Check sheet for the modelled part. Datum: model origin and axes. Units: mm. Round coordinates to 2 decimals unless told otherwise and drop trailing zeros. Order: outer loops, then holes, each group sorted by start corner. A loop starts at its lowest first (then second) coordinate and runs counter-clockwise, first axis right, second up. Notation, with made-up numbers: (-38, 20) -> (-29, 20) arc R18 cw to (-29, 52) -> close; hole circle Ø9 at (-9, 4). An arc over 180 degrees is marked (long way). Answer in a Markdown table with one row per item.
from build123d import *

# Parameters (mm, degrees)
F1_DEPTH = 8


with BuildPart() as f1:
    # F0 (on Top) → F1 (new body)
    with BuildSketch(Plane.XY):
        with BuildLine():
            Line((24.033267, 22.719095), (12.033267, 22.719095))
            ThreePointArc((12.033267, 22.719095), (10.619054, 22.133308), (10.033267, 20.719095))
            Line((10.033267, 20.719095), (10.033267, 9.719095))
            ThreePointArc((10.033267, 9.719095), (10.619054, 8.304881), (12.033267, 7.719095))
            Line((12.033267, 7.719095), (24.033267, 7.719095))
            ThreePointArc((24.033267, 7.719095), (25.447481, 8.304881), (26.033267, 9.719095))
            Line((26.033267, 9.719095), (26.033267, 20.719095))
            ThreePointArc((26.033267, 20.719095), (25.447481, 22.133308), (24.033267, 22.719095))
        make_face()
        with BuildLine():
            ThreePointArc((20.633267, 11.719095), (16.19479, 9.880617), (18.033267, 14.319095))
            ThreePointArc((18.033267, 14.319095), (19.871745, 13.557572), (20.633267, 11.719095))
        make_face(mode=Mode.SUBTRACT)
        with BuildLine():
            ThreePointArc((18.033267, 16.119095), (16.19479, 20.557572), (20.633267, 18.719095))
            ThreePointArc((20.633267, 18.719095), (19.871745, 16.880617), (18.033267, 16.119095))
        make_face(mode=Mode.SUBTRACT)
    extrude(amount=F1_DEPTH)


solid = f1.part
Item 1: Cross-section at A-A (z = 7.5). Record the boundary of the cut face in (x, y), and give its area (3 significant figures).
Result sheet:
| item | result |
|---|---|
| outline | (10.03, 9.72) arc R2 ccw to (12.03, 7.72) -> (24.03, 7.72) arc R2 ccw to (26.03, 9.72) -> (26.03, 20.72) arc R2 ccw to (24.03, 22.72) -> (12.03, 22.72) arc R2 ccw to (10.03, 20.72) -> close; hole circle Ø5.2 at (18.03, 11.72); hole circle Ø5.2 at (18.03, 18.72) |
| area | 194 mm^2 |
Item 2: Cross-section at C-C (y = 12.75). Record the boundary of the cut face in (x, z), and give its area (3 significant figures).
Result sheet:
| item | result |
|---|---|
| outline | (10.03, 0) -> (15.65, 0) -> (15.65, 8) -> (10.03, 8) -> close; (20.42, 0) -> (26.03, 0) -> (26.03, 8) -> (20.42, 8) -> close |
| area | 89.8 mm^2 |
Item 3: Cross-section at B-B (x = 17.5). Record the boundary of the cut face in (y, z).
Result sheet:
| item | result |
|---|---|
| outline | (7.72, 0) -> (9.17, 0) -> (9.17, 8) -> (7.72, 8) -> close; (14.26, 0) -> (16.17, 0) -> (16.17, 8) -> (14.26, 8) -> close; (21.26, 0) -> (22.72, 0) -> (22.72, 8) -> (21.26, 8) -> close |
Item 4: Scan lines: line 1 (Y direction, x = 19.5, z = 4); line 2 (X direction, y = 12.75, z = 4); line 3 (Y direction, x = 20, z = 1). Record each from-to range of solid material in increasing order. Write a range as [from, to].
Result sheet:
| item | result |
|---|---|
| line 1 | y = [7.72, 9.57], [13.87, 16.57], [20.87, 22.72] |
| line 2 | x = [10.03, 15.65], [20.42, 26.03] |
| line 3 | y = [7.72, 10.02], [13.42, 17.02], [20.42, 22.72] |
Item 5: Depth check by flat-ended pin: P1, Ø4, axis at x = 18.03, y = 18.72, coming from the +Z side. Enter the tip coordinate at first touch or a pass-through.
Result sheet:
| item | result |
|---|---|
| P1 | passes through |
Item 6: Cross-section at D-D (y = 8.5). Record the boundary of the cut face in (x, z), and give its area (3 significant figures).
Result sheet:
| item | result |
|---|---|
| outline | (10.45, 0) -> (25.62, 0) -> (25.62, 8) -> (10.45, 8) -> close |
| area | 121 mm^2 |
